Autodesk Inventor part; units mm, degrees
ref_plane "YZ Plane" through (0, 0, 0) normal (1, 0, 0) x (0, 1, 0)
ref_plane "XZ Plane" through (0, 0, 0) normal (0, 1, 0) x (-1, 0, 0)
ref_plane "XY Plane" through (0, 0, 0) normal (0, 0, 1) x (1, 0, 0)
sketch "スケッチ2" plane through (0, 0, 0) normal (1, 0, 0) x (0, 1, 0)
  line L0 (0, 0) -> (5, 0)
  line L1 (5, 0) -> (5, -75)
  line L2 (5, -75) -> (0, -75)
  line L3 (0, -75) -> (0, 0)
  line L4 (0, 0) -> (-70, 0)
  line L5 (-70, 0) -> (-70, -5)
  line L6 (-70, -5) -> (0, -5)
  line L7 (0, -5) -> (0, 0)
  point P0 (-70, -2.5)
  point P1 (0, -5)
  dimension "d0" = 75
  dimension "d1" = 75
  dimension "d2" = 5
  dimension "d3" = 5
extrude "押し出し1" add sketch "スケッチ2" along normal blind 75
sketch "スケッチ4" plane through (75, 0, 0) normal (1, 0, 0) x (0, 0, -1)
  line L0 (0, 0) -> (13, 0)
  line L1 (0, 0) -> (5, 0)
  line L2 (75, 5) -> (0, 5)
  line L3 (0, 5) -> (0, -70)
  circle A0 centre (2.5, 2.5) radius 10
  dimension "d32" = 2.5
  dimension "d33" = 2.5
  dimension "d34" = 20
extrude "押し出し2" add sketch "スケッチ4" along normal blind 5
sketch "スケッチ7" plane through (80, 2.5, -2.5) normal (1, 0, 0) x (0, 0, -1)
  point P0 (-2.5, -2.5)
  point P1 (0, 7)
  point P2 (-7, 0)
  point P3 (0, 0)
  dimension "d35" = 7
  dimension "d36" = 7
hole "穴2" at (80, 9.5, -2.5) at (80, 2.5, 4.5) direction (-1, 0, 0) diameter 2 depth 8.1 tip angle 118
properties part number "排出機構"
The model under review builds one solid part; all positions refer to its coordinate system, in mm. A direction names the side the tool comes from. Coordinates: 2 decimals unless noted, no trailing zeros. Write each loop counter-clockwise with the first axis right and the second up, starting at its lowest first coordinate (ties: lowest second). Pieces come first, ordered by that corner, then holes. Notation, with made-up numbers: (-25, 60.5) - (-6, 60.5) arc R20 ccw to (-6, 76.5) - close; hole circle Ø9 at (-22.75, -23). An arc over 180 degrees is marked (long way). Answer in a Markdown table with one row per item. Add a question column.
Q1. Consider section B-B on y = -4. Give the boundary of the cut face in (x, z).
Q2. Consider section D-D on y = -43.5. Give the boundary of the cut face in (x, z), then the cut area to 3 significant figures.
Q3. For faces 1 (the face through (75, 2, -43)), 2 (the face through (80, 3, -2)), 3 (the face through (75, -3, -8)), 4 (the face through (37, 5, -37)), 5 (the face through (75, -39, -2)), list the 3-axis set-ups (+Z, -Z, +X, -X, +Y, -Y) from which the entire face can be reached by the end or side of a thin tool; tool diameter is ignored.
Q4. To check wall thickness, follow line 1 along Z through (x, y) = (78.9, 2.5); line 2 along Y through (x, z) = (76.6, -2.5); line 3 along X through (y, z) = (5.5, -8). State the ranges of each line that lie inside material, in increasing order. Write a range as from..to.
Q5. Consider section C-C on z = -53. Give the boundary of the cut face in (x, y).
Q6. Clearance check with flat-ended pins moving along their axes: pin 1 (2.5 mm diameter, centred on y = -24.5, z = -1.5, fed in from +X); pin 2 (10 mm diameter, centred on x = 61.5, z = -51, fed in from +Y); pin 3 (21 mm diameter, centred on x = 31, z = -45, fed in from -Y). State where each tip first meets the part, or that it passes through.
Q7. Consider section A-A on x = 57. Give the boundary of the cut face in (y, z).
Answers below:
| question | item | result |
|---|---|---|
| 1 | outline | (0, -5) - (75, -5) - (75, -10.1) - (80, -10.1) - (80, 5.1) - (75, 5.1) - (75, 0) - (0, 0) - close |
| 2 | outline | (0, -5) - (75, -5) - (75, 0) - (0, 0) - close |
| 2 | area | 375 mm² |
| 3 | face 1 | -Z, +X, +Y, -Y |
| 3 | face 2 | +Z, -Z, +X, +Y, -Y |
| 3 | face 3 | -Z, -X, -Y |
| 3 | face 4 | +Z, -Z, -X, +Y |
| 3 | face 5 | +Z, -Z, +X, -Y |
| 4 | line 1 | -12.5..3.5, 5.5..7.5 |
| 4 | line 2 | -7.5..8.5, 10.5..12.5 |
| 4 | line 3 | 75..80 |
| 5 | outline | (0, 0) - (75, 0) - (75, 5) - (0, 5) - close |
| 6 | pin 1 | x = 75 |
| 6 | pin 2 | y = 5 |
| 6 | pin 3 | y = 0 |
| 7 | outline | (-70, -5) - (0, -5) - (0, -75) - (5, -75) - (5, 0) - (-70, 0) - close |
